Autodesk Inventor part; units mm, degrees
ref_plane "to_screw1_XY" through (10, -2.8284, 2.8284) normal (0, -0.7071068, 0.7071068) x (1, 0, 0)
ref_plane "to_screw1_YZ" through (10, -2.8284, 2.8284) normal (1, 0, 0) x (0, 0.7071068, 0.7071068)
ref_plane "to_screw1_ZX" through (10, -2.8284, 2.8284) normal (0, 0.7071068, 0.7071068) x (0, -0.7071068, 0.7071068)
sketch "Sketch_1" plane through (0, 0, 0) normal (0, 0, 1) x (1, 0, 0)
  line L0 (16, 0) -> (0, 0)
  line L1 (0, 4) -> (16, 4)
  line L2 (16, 4) -> (16, 6)
  line L3 (16, 6) -> (5, 6)
  line L4 (5, 6) -> (5, 14)
  line L5 (5, 14) -> (0, 14)
  line L6 (0, 14) -> (0, 4)
revolve "Revolution1" add sketch "Sketch_1" angle 360 about axis through (16, 0, 0) along (1, 0, 0)
sketch "Sketch_19" plane through (10, 0, 0) normal (1, 0, 0) x (0, 0, -1)
  line L0 (-2.1213, 2.1213) -> (-4.2426, 4.2426)
  line L1 (-4.2426, 4.2426) -> (-3.182, 5.3033)
  line L2 (-3.182, 5.3033) -> (-3.182, 4.9208)
  line L3 (-3.182, 4.9208) -> (-1.2519, 2.9907)
  line L4 (-1.2519, 2.9907) -> (-2.1213, 2.1213)
  line L5 (-2.1213, 2.1213) -> (-4.2426, 4.2426)
revolve "Revolution2" cut sketch "Sketch_19" angle 360 about axis through (10, 2.1213, 2.1213) along (0, -0.7071068, -0.7071068)
thread "Thread1"
sketch "Sketch_3" plane through (10, 0, 0) normal (1, 0, 0) x (0, 0, -1)
  line L0 (-2.1213, -2.1213) -> (-4.2426, -4.2426)
  line L1 (-4.2426, -4.2426) -> (-5.3033, -3.182)
  line L2 (-5.3033, -3.182) -> (-4.9208, -3.182)
  line L3 (-4.9208, -3.182) -> (-2.9907, -1.2519)
  line L4 (-2.9907, -1.2519) -> (-2.1213, -2.1213)
  line L5 (-2.1213, -2.1213) -> (-4.2426, -4.2426)
revolve "Revolution3" cut sketch "Sketch_3" angle 360 about axis through (10, -2.1213, 2.1213) along (0, 0.7071068, -0.7071068)
thread "Thread2"
sketch "Sketch4" plane through (5, 0, 0) normal (1, 0, 0) x (0, 0, -1)
  point P0 (0, 10)
hole "Hole1" at (5, 10, 0) direction (-1, 0, 0) diameter 3.5 depth 5
sketch "Sketch5" plane through (0, 0, 0) normal (-1, 0, 0) x (0, 0, 1)
  point P0 (0, -10)
hole "Hole2" at (0, -10, 0) direction (1, 0, 0) diameter 3.5 depth 5
sketch "Sketch_4" plane through (0, 0, 0) normal (1, 0, 0) x (0, 1, 0)
  circle A0 centre (0, 0) radius 150
  line L0 (50, 8) -> (-50, 8)
  line L1 (-50, 8) -> (-50, -8)
  line L2 (-50, -8) -> (50, -8)
  line L3 (50, -8) -> (50, 8)
extrude "Extrusion1" cut sketch "Sketch_4" along normal blind 16
ref_plane "to_screw1_XY" through (10, -2.8284, 2.8284) normal (0, -0.7071068, 0.7071068) x (1, 0, 0)
ref_plane "to_screw1_YZ" through (10, -2.8284, 2.8284) normal (1, 0, 0) x (0, 0.7071068, 0.7071068)
ref_plane "to_screw1_ZX" through (10, -2.8284, 2.8284) normal (0, 0.7071068, 0.7071068) x (0, -0.7071068, 0.7071068)
ref_plane "to_screw2_XY" through (10, 2.8284, 2.8284) normal (0, 0.7071068, 0.7071068) x (1, 0, 0)
ref_plane "to_screw2_YZ" through (10, 2.8284, 2.8284) normal (1, 0, 0) x (0, 0.7071068, -0.7071068)
ref_plane "to_screw2_ZX" through (10, 2.8284, 2.8284) normal (0, 0.7071068, -0.7071068) x (0, 0.7071068, 0.7071068)
properties part number "ATHC8-MB_b"
Source: CAD feature listing. Evaluate the final solid. Frame: model axes, mm. Give positions to 0.01 mm unless a question says otherwise; leave off trailing zeros. Loops run counter-clockwise (first coordinate to the right, second up) from the corner with the lowest first, then second, coordinate; pieces in that order, holes last. Notation, with made-up numbers: M 18.5,57.5 L 24.5,57.5 A20 cw 24.5,65.5 Z; hole C -15.5,-16 d11. An arc over 180 degrees is marked long. Put each result on its own line as item: value.
Q1. Section D-D (y = 10). Return the cut outline in (x, z), and give its area (3 significant figures).
Response values:
outline: M 0,-8 L 5,-8 L 5,-1.75 L 0,-1.75 Z; M 0,1.75 L 5,1.75 L 5,8 L 0,8 Z
area: 62.5 mm²
Q2. Section A-A (y = 0). Return the cut outline in (x, z).
Response values:
outline: M 0,-8 L 5,-8 L 5,-6 L 16,-6 L 16,-4 L 0,-4 Z; M 0,4 L 16,4 L 16,6 L 5,6 L 5,8 L 0,8 Z
Q3. Line query: probe 1 along Z at (x, y) = (3.85, -10); probe 2 along Y at (x, z) = (1.5, 0.5); probe 3 along X at (y, z) = (10.25, -4.5). Output: solid intervals per line, ascending. Write a range as [from, to].
Response values:
probe 1: z = [-8, -1.75], [1.75, 8]
probe 2: y = [-13.99, -11.68], [-8.32, -3.97], [3.97, 8.32], [11.68, 13.99]
probe 3: x = [0, 5]
Q4. Section B-B (z = 0). Return the cut outline in (x, y).
Response values:
outline: M 0,-14 L 5,-14 L 5,-11.75 L 0,-11.75 Z; M 0,-8.25 L 5,-8.25 L 5,-6 L 16,-6 L 16,-4 L 0,-4 Z; M 0,4 L 16,4 L 16,6 L 5,6 L 5,8.25 L 0,8.25 Z; M 0,11.75 L 5,11.75 L 5,14 L 0,14 Z
Q5. Pin query (flat end, axial travel): P1, Ø6, axis at x = 13.5, y = 9.5, coming from the +Z side; P2, Ø5, axis at x = 7, y = -2.5, coming from the -Z side; P3, Ø4.5, axis at y = 10, z = 0, coming from the +X side. Return the tip coordinate at first contact, or that it passes through.
Response values:
P1: passes through
P2: stops at z = -8
P3: stops at x = 5
Q6. Section C-C (x = 5.5). Return the cut outline in (y, z), and give its area (3 significant figures).
Response values:
outline: C 0,0 d12; hole C 0,0 d8
area: 62.8 mm²
Q7. Mould query, pull axis Y, two halves, no side actions, for faces 1 (the cylindrical face through (10.05, 2.49, 4.23)), 2 (the flat face through (2, 0, -8)), 3 (the cylindrical face through (10.423, 5.723, -1.802)). Classes: released by +Y, released by -Y, zero draft, split by the parting line, or undercut.
Response values:
face 1: undercut
face 2: zero draft
face 3: split by the parting line
